Work out the finished part from the listing and answer in its coordinate system (mm). Face numbers are marked on the shaded views. Give positions to 0.01 mm unless a question says otherwise; leave off trailing zeros. Loops run counter-clockwise (first coordinate to the right, second up) from the corner with the lowest first, then second, coordinate; pieces in that order, holes last. Notation, with made-up numbers: M 63.25,25 L 95.25,25 A18 ccw 95.25,36 Z; hole C 25,63 d5. An arc over 180 degrees is marked long. Answer in a Markdown table with one row per item. Add a question column.
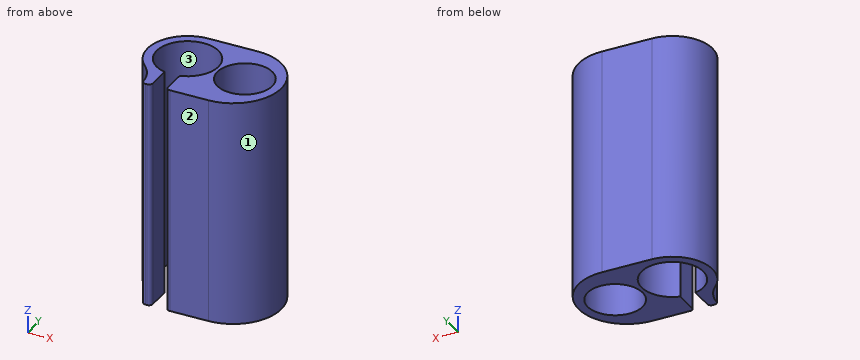
from build123d import *

# Parameters (mm, degrees)
BOSS_EXTRU_1_DEPTH      = 60
ESQUISSE2_R             = 7.25
ENL_V_MAT_EXTRU_1_DEPTH = 61
CONG_1_R                = 10
CONG_2_R                = 1


with BuildPart() as part:
    # Esquisse1 → Boss.-Extru.1 (new body)
    with BuildSketch(Plane.XY):
        with BuildLine():
            Line((-2, -7.9007911), (-2, -14.9007911))
            Line((-2, -14.9007911), (-4.4, -14.9007911))
            Line((-4.4, -14.9007911), (-4.4, -9.588665183))
            ThreePointArc((-4.4, -9.588665183), (-10.306864647, 2.251897235), (0, 10.55))
            Line((0, 10.55), (13.147142873, 10.55))
            ThreePointArc((13.147142873, 10.55), (25.872538423, -2.17539555), (13.147142873, -14.9007911))
            Line((13.147142873, -14.9007911), (4.4, -14.9007911))
            Line((4.4, -14.9007911), (2, -14.9007911))
            Line((2, -14.9007911), (2, -7.9007911))
            ThreePointArc((2, -7.9007911), (0, 8.15), (-2, -7.9007911))
        make_face()
    extrude(amount=BOSS_EXTRU_1_DEPTH)

    # Esquisse2 → Enlèv. mat.-Extru.1 (cut, through all)
    with BuildSketch(Plane(origin=(0, 0, 0), x_dir=(-1, 0, 0), z_dir=(0, 0, -1))):
        with Locations((-16.23903239, -2.17539555)):
            Circle(ESQUISSE2_R)
    extrude(amount=-ENL_V_MAT_EXTRU_1_DEPTH, mode=Mode.SUBTRACT)

    # Congé1
    cong_1_edges = [part.edges().sort_by_distance(p)[0] for p in [
        (-4.4, -9.588665183, 30),
    ]]
    fillet(cong_1_edges, radius=CONG_1_R)

    # Congé2
    cong_2_edges = [part.edges().sort_by_distance(p)[0] for p in [
        (-4.4, -14.9007911, 30),
        (-2, -14.9007911, 30),
        (2, -14.9007911, 30),
    ]]
    fillet(cong_2_edges, radius=CONG_2_R)


solid = part.part
(1) Section A-A, the plane y = -3.25 is taken. Determine the outline of the cut face in (x, z), and give its area (3 significant figures).
(2) The mould has two halves that part along X. Classify the marked faces 1, 2 and 3: pulls with the +X half, pulls with the -X half, needs draft (parallel to the pull), parting line crosses it, or undercut.
(3) Section B-B, the plane y = -11.5 is taken. Determine the outline of the cut face in (x, z), and give its area (3 significant figures).
(4) Section C-C, the plane y = 0 is taken. Determine the outline of the cut face in (x, z), and give its area (3 significant figures).
(5) Consider line 1 along X through (y, z) = (2, 12.5); line 2 along X through (y, z) = (0, 22); line 3 along X through (y, z) = (-13.5, 13). Determine where each line is inside the solid, lowest interval first. Write a range as from..to.
(6) Each of these flat-tipped pins is pushed along its axis until it touches: P1, Ø1.5, axis at y = -1.5, z = 37, coming from the -X side; P2, Ø6, axis at y = -9, z = 25.5, coming from the +X side; P3, Ø1.8, axis at y = -12, z = 35, coming from the +X side. Where does it stop, or does it pass through?
(7) Section D-D, the plane y = 6 is taken. Determine the outline of the cut face in (x, z).
Numbers:
| question | item | result |
|---|---|---|
| 1 | outline | M -10.04,0 L -7.47,0 L -7.47,60 L -10.04,60 Z; M 7.47,0 L 9.07,0 L 9.07,60 L 7.47,60 Z; M 23.41,0 L 25.83,0 L 25.83,60 L 23.41,60 Z |
| 1 | area | 395 mm² |
| 2 | face 1 | pulls with the +X half |
| 2 | face 2 | needs draft |
| 2 | face 3 | undercut |
| 3 | outline | M -4.91,0 L -2,0 L -2,60 L -4.91,60 Z; M 2,0 L 21.81,0 L 21.81,60 L 2,60 Z |
| 3 | area | 1,360 mm² |
| 4 | outline | M -10.55,0 L -8.15,0 L -8.15,60 L -10.55,60 Z; M 8.15,0 L 9.32,0 L 9.32,60 L 8.15,60 Z; M 23.15,0 L 25.69,0 L 25.69,60 L 23.15,60 Z |
| 4 | area | 366 mm² |
| 5 | line 1 | x = -10.36..-7.9, 7.9..10.31, 22.17..25.17 |
| 5 | line 2 | x = -10.55..-8.15, 8.15..9.32, 23.15..25.69 |
| 5 | line 3 | x = -4.47..-2, 2..18.95 |
| 6 | P1 | stops at x = -10.52 |
| 6 | P2 | stops at x = 25.28 |
| 6 | P3 | stops at x = 22.22 |
| 7 | outline | M -8.68,0 L -5.52,0 L -5.52,60 L -8.68,60 Z; M 5.52,0 L 22.9,0 L 22.9,60 L 5.52,60 Z |
